```python
from build123d import *

# Parameters (mm, degrees)
SKETCH1_R         = 7.25
FLANGE_DEPTH      = 2.5
BARREL_START      = 2.5
SKETCH2_R         = 4.75
BARREL_DEPTH      = 12
REAR_THREAD_START = -8
SKETCH3_R         = 4.75
REAR_THREAD_DEPTH = 8
REAR_NUT_START    = -5.5
SKETCH4_R         = 6.25
REAR_NUT_DEPTH    = 2.5
SOCKET_BORE_START = 14.5
SKETCH5_R         = 3.25
SOCKET_BORE_DEPTH = 8


with BuildPart() as part:
    # Sketch1 → Flange (new body)
    with BuildSketch(Plane.XY):
        Circle(SKETCH1_R)
    extrude(amount=FLANGE_DEPTH)

    # Sketch2 → Barrel (add)
    with BuildSketch(Plane.XY.offset(BARREL_START)):
        Circle(SKETCH2_R)
    extrude(amount=BARREL_DEPTH)

    # Sketch3 → Rear_Thread (add)
    with BuildSketch(Plane.XY.offset(REAR_THREAD_START)):
        Circle(SKETCH3_R)
    extrude(amount=REAR_THREAD_DEPTH)

    # Sketch4 → Rear_Nut (add)
    with BuildSketch(Plane.XY.offset(REAR_NUT_START)):
        Circle(SKETCH4_R)
    extrude(amount=REAR_NUT_DEPTH)

    # Sketch5 → Socket_Bore (cut)
    with BuildSketch(Plane.XY.offset(SOCKET_BORE_START)):
        Circle(SKETCH5_R)
    extrude(amount=-SOCKET_BORE_DEPTH, mode=Mode.SUBTRACT)


solid = part.part
```
Check sheet for the modelled part. Datum: model origin and axes. Units: mm. A direction names the side the tool comes from. Round coordinates to 2 decimals unless told otherwise and drop trailing zeros. Order: outer loops, then holes, each group sorted by start corner. A loop starts at its lowest first (then second) coordinate and runs counter-clockwise, first axis right, second up. Notation, with made-up numbers: (4, 81.5) - (27, 81.5) arc R9 cw to (27, 95.5) - close; hole circle Ø11 at (-12.75, -16.5). An arc over 180 degrees is marked (long way). Write item = value, one per line.
Q1. Tool access check on faces 4 (the face through (2, -3, 14.5)), 5 (the face through (2.192, -4.214, -6.768)), 6 (the face through (3.35, -6.43, 1.23)), 7 (the face through (2.192, -4.214, 8.416)), 8 (the face through (2, -5, 0)). Record the directions out of +Z, -Z, +X, -X, +Y, -Y that give a thin tool (end or side, any length) a straight path to the whole face; none if there is none.
Computed:
face_4 = +Z, +X, -X, +Y, -Y
face_5 = -Z
face_6 = +Z, -Z
face_7 = +Z
face_8 = none
Q2. Thickness scan on line 1 along Z through (x, y) = (-5, 3.25); line 2 along Y through (x, z) = (0, 9.25); line 3 along Z through (x, y) = (2, -0.75). Record the ranges inside material, lowest first.
Computed:
line_1 = -5.5 to -3, 0 to 2.5
line_2 = -4.75 to -3.25, 3.25 to 4.75
line_3 = -8 to 6.5
Q3. Section check D-D (z = 13.25). Record the boundary of the cut face in (x, y), and give its area (3 significant figures).
Computed:
outline = circle Ø9.5 at (0, 0); hole circle Ø6.5 at (0, 0)
area = 37.7 mm^2
Q4. Go/stop test with flat-tipped pins: pin 1 (2 mm diameter, centred on x = -0.5, y = 1.5, fed in from +Z); pin 2 (2 mm diameter, centred on y = 2.5, z = 10.5, fed in from +X); pin 3 (3 mm diameter, centred on x = 1.5, z = 5.5, fed in from +Y). Record where each tip stops, or that it passes through.
Computed:
pin_1 = 6.5
pin_2 = 4.51
pin_3 = 4.75
Q5. Draft check along X on faces 1 (the face through (-2.579, -1.978, 10.556)), 2 (the face through (2.192, -4.214, -1.521)), 3 (the face through (-1, 5, -3)). Enter one of: pulls with the +X half, pulls with the -X half, needs draft (parallel to the pull), parting line crosses it, or undercut.
Computed:
face_1 = undercut
face_2 = parting line crosses it
face_3 = needs draft
Q6. Section check C-C (x = 5.5). Record the boundary of the cut face in (y, z), and give its area (3 significant figures).
Computed:
outline = (-4.72, 0) - (4.72, 0) - (4.72, 2.5) - (-4.72, 2.5) - close; (-2.97, -5.5) - (2.97, -5.5) - (2.97, -3) - (-2.97, -3) - close
area = 38.5 mm^2
Q7. Section check A-A (x = 0). Record the boundary of the cut face in (y, z).
Computed:
outline = (-7.25, 0) - (-4.75, 0) - (-4.75, -3) - (-6.25, -3) - (-6.25, -5.5) - (-4.75, -5.5) - (-4.75, -8) - (4.75, -8) - (4.75, -5.5) - (6.25, -5.5) - (6.25, -3) - (4.75, -3) - (4.75, 0) - (7.25, 0) - (7.25, 2.5) - (4.75, 2.5) - (4.75, 14.5) - (3.25, 14.5) - (3.25, 6.5) - (-3.25, 6.5) - (-3.25, 14.5) - (-4.75, 14.5) - (-4.75, 2.5) - (-7.25, 2.5) - close
Q8. Section check B-B (y = -1). Record the boundary of the cut face in (x, z).
Computed:
outline = (-7.18, 0) - (-4.64, 0) - (-4.64, -3) - (-6.17, -3) - (-6.17, -5.5) - (-4.64, -5.5) - (-4.64, -8) - (4.64, -8) - (4.64, -5.5) - (6.17, -5.5) - (6.17, -3) - (4.64, -3) - (4.64, 0) - (7.18, 0) - (7.18, 2.5) - (4.64, 2.5) - (4.64, 14.5) - (3.09, 14.5) - (3.09, 6.5) - (-3.09, 6.5) - (-3.09, 14.5) - (-4.64, 14.5) - (-4.64, 2.5) - (-7.18, 2.5) - close
